Check sheet for the drawn part. Datum: minimum x, y, z corner. Units: mm. A direction names the side the tool comes from. Coordinates: 2 decimals unless noted, no trailing zeros. Write each loop counter-clockwise with the first axis right and the second up, starting at its lowest first coordinate (ties: lowest second). Pieces come first, ordered by that corner, then holes. Notation, with made-up numbers: M 79.25,30 L 113.25,30 A15 ccw 113.25,49 Z; hole C -15,-30.5 d11. An arc over 180 degrees is marked long. Answer as CSV lines item,"result". Start each with the question number.
Q1. Access from +Z, -Z, +X, -X, +Y, -Y to the whole of each face (thin tool, end or side, straight path). Record for the marked faces 1 and 2.
Q2. Sectioned sample at D-D, the plane z = 31. Record the cut outline in (x, y).
Q3. Sectioned sample at A-A, the plane x = 32.5. Record the cut outline in (y, z), then the cut area to 3 significant figures.
Q4. Sectioned sample at C-C, the plane x = 48.5. Record the cut outline in (y, z), then the cut area to 3 significant figures.
Q5. Sectioned sample at B-B, the plane y = 17.5. Record the cut outline in (x, z), then the cut area to 4 significant figures.
Q6. Thickness scan on line 1 along X through (y, z) = (36.5, 68); line 2 along Z through (x, y) = (32, 24); line 3 along Z through (x, y) = (32, 36). Record the ranges inside material, lowest first. Write a range as from..to.
Q7. Mould release check, pull along Z, two halves, no side actions. Record for the marked faces 3, 4 and 5: pulls with the +Z half, pulls with the -Z half, needs draft (parallel to the pull), parting line crosses it, or undercut.
Q8. Depth check by flat-ended pin: pin 1 Ø2 at (x, z) = (23.5, 25) entering from +Y; pin 2 Ø6 at (x, z) = (27, 87) entering from -Y; pin 3 Ø4.5 at (x, y) = (30, 6.5) entering from +Z. Enter the tip coordinate at first touch or a pass-through.
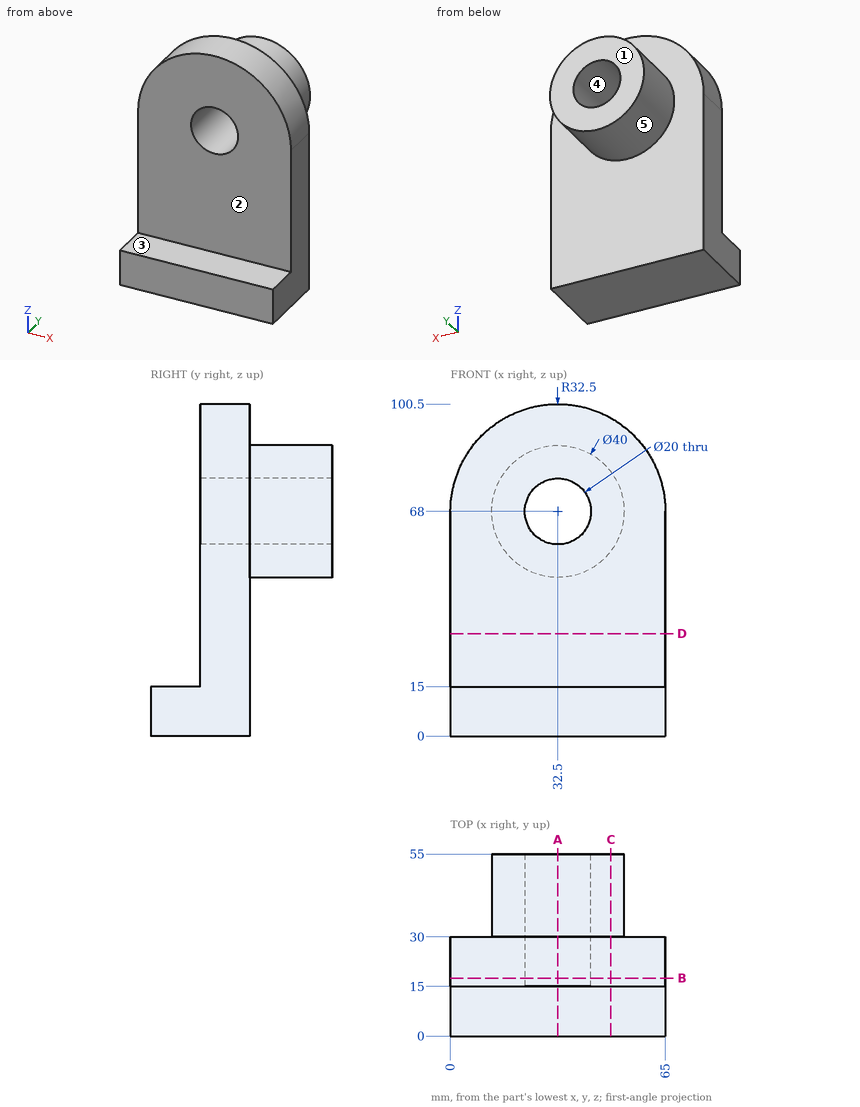
Output:
1,face 1,"+Z, -Z, +X, -X, +Y"
1,face 2,"+Z, +X, -X, -Y"
2,outline,"M 0,15 L 65,15 L 65,30 L 0,30 Z"
3,outline,"M 0,0 L 30,0 L 30,48 L 55,48 L 55,58 L 15,58 L 15,15 L 0,15 Z; M 15,78 L 55,78 L 55,88 L 30,88 L 30,100.5 L 15,100.5 Z"
3,area,"1,930 mm^2"
4,outline,"M 0,0 L 30,0 L 30,56 L 55,56 L 55,80 L 30,80 L 30,96.29 L 15,96.29 L 15,15 L 0,15 Z"
4,area,"2,270 mm^2"
5,outline,"M 0,0 L 65,0 L 65,68 A32.5 ccw 0,68 Z; hole C 32.5,68 d20"
5,area,"5,765 mm^2"
6,line 1,"x = 12.5..22.5, 42.5..52.5"
6,line 2,"z = 0..58.01, 77.99..100.5"
6,line 3,"z = 48.01..58.01, 77.99..87.99"
7,face 3,"pulls with the +Z half"
7,face 4,"undercut"
7,face 5,"parting line crosses it"
8,pin 1,"stops at y = 30"
8,pin 2,"stops at y = 15"
8,pin 3,"stops at z = 15"
